Autodesk Inventor part; units mm, degrees
ref_plane "YZ Plane" through (0, 0, 0) normal (1, 0, 0) x (0, 1, 0)
ref_plane "XZ Plane" through (0, 0, 0) normal (0, 1, 0) x (-1, 0, 0)
ref_plane "XY Plane" through (0, 0, 0) normal (0, 0, 1) x (1, 0, 0)
sketch "Sketch1" plane through (0, 0, 0) normal (0, 0, 1) x (1, 0, 0)
  circle A0 centre (0, 0) radius 75.5
  dimension "d0" = 151
extrude "Extrusion1" add sketch "Sketch1" against normal blind 5
sketch "Sketch2" plane through (0, 0, 0) normal (0, 0, 1) x (1, 0, 0)
  circle A0 centre (0, 0) radius 71.5 construction
  point P0 (0, 71.5)
  dimension "d3" = 143
hole "Hole1" at (0, 71.5, 0) direction (0, 0, -1) diameter 5 depth 5
pattern_circular "Circular Pattern1" count 12 over 360 about axis through (0, 0, 0) along (0, 0, -1) of "Hole1"
fillet "Fillet1" radius 0.5 2 edges at (-75.5, 0, 0) (-75.5, 0, -5)
properties part number "101 part 1" material "Silver"
For this review, take the finished solid that the model builds, in its own axes (mm). Round coordinates to 2 decimals unless told otherwise and drop trailing zeros. Write each loop counter-clockwise with the first axis right and the second up, starting at its lowest first coordinate (ties: lowest second). Pieces come first, ordered by that corner, then holes. Notation, with made-up numbers: (86, -31) - (97, -31) arc R21 cw to (97, 4) - close; hole circle Ø5 at (68, 39). An arc over 180 degrees is marked (long way). Use a Markdown table: item, result.
Q1. We need section A-A (y = 0). Give the boundary of the cut face in (x, z).
Derived:
| item | result |
|---|---|
| outline | (-75.5, -4.5) arc R0.5 ccw to (-75, -5) - (-74, -5) - (-74, 0) - (-75, 0) arc R0.5 ccw to (-75.5, -0.5) - close; (-69, -5) - (69, -5) - (69, 0) - (-69, 0) - close; (74, -5) - (75, -5) arc R0.5 ccw to (75.5, -4.5) - (75.5, -0.5) arc R0.5 ccw to (75, 0) - (74, 0) - close |
Q2. We need section C-C (z = -2.85). State how many separate pieces and enclosed holes the cut face has, plus the area to 3 significant figures.
Derived:
| item | result |
|---|---|
| separate pieces | 1 |
| enclosed holes | 12 |
| area | 17,700 mm2 |
Q3. Wall thickness on line 1 along Y through (x, z) = (1.5, -2.5); line 2 along Y through (x, z) = (-0.5, -1); line 3 along X through (y, z) = (63.5, -1.1): over which ranges is each line inside the solid? List them lowest first.
Derived:
| item | result |
|---|---|
| line 1 | y = -75.49 to -73.5, -69.5 to 69.5, 73.5 to 75.49 |
| line 2 | y = -75.5 to -73.95, -69.05 to 69.05, 73.95 to 75.5 |
| line 3 | x = -40.84 to -37.69, -33.81 to 33.81, 37.69 to 40.84 |
Q4. The part is to be moulded in two halves that separate along X. For faces 1 (the cylindrical face through (72.014, 22.678, -2.472)), 2 (the cylindrical face through (74, 0, -3)), 3 (the flat face through (-1, 1, -5)), say which applies: pulls with the +X half, pulls with the -X half, needs draft (parallel to the pull), parting line crosses it, or undercut.
Derived:
| item | result |
|---|---|
| face 1 | parting line crosses it |
| face 2 | undercut |
| face 3 | needs draft |
Q5. Clearance check with flat-ended pins moving along their axes: pin 1 (10 mm diameter, centred on x = -50, y = 10.5, fed in from +Z); pin 2 (2 mm diameter, centred on y = -38.5, z = -3.5, fed in from +X); pin 3 (1.5 mm diameter, centred on x = -11.5, z = -1, fed in from -Y); pin 4 (1.5 mm diameter, centred on x = -54, z = -0.5, fed in from -Y). State where each tip first meets the part, or that it passes through.
Derived:
| item | result |
|---|---|
| pin 1 | stops at z = 0 |
| pin 2 | stops at x = 65.53 |
| pin 3 | stops at y = -74.73 |
| pin 4 | stops at y = -53.52 |
